Geometry: final body of the model. Coordinates: model frame, mm. A direction names the side the tool comes from. Coordinates: 2 decimals unless noted, no trailing zeros. One line per item, written item: value.
```python
from build123d import *

# Parameters (mm, degrees)
F1_DEPTH = 18
F3_D     = 3
F3_DEPTH = 17.5
F3_TIP   = 0.9012909285
F5_D     = 3
F5_DEPTH = 17.5
F5_TIP   = 0.9012909285
F7_D     = 3
F7_DEPTH = 17.5
F7_TIP   = 0.9012909285


with BuildPart() as f1:
    # F0 (on Top) → F1 (new body)
    with BuildSketch(Plane.XY):
        Polygon((65, 65), (55, 65), (-55, 65), (-65, 65), (-65, 55), (-65, -55), (-65, -65), (-55, -65), (55, -65), (65, -65), (65, -55), (65, 55), align=None)
    extrude(amount=F1_DEPTH)

    # F3
    with Locations(Plane.XZ.offset(65)):
        with Locations((0, 9)):
            Hole(F3_D / 2, depth=F3_DEPTH)
            with Locations((0, 0, -(F3_DEPTH + F3_TIP / 2))):  # 118° drill point
                Cone(0, F3_D / 2, F3_TIP, mode=Mode.SUBTRACT)

    # F5
    with Locations(Plane.YZ.offset(65)):
        with Locations((42.5, 9)):
            Hole(F5_D / 2, depth=F5_DEPTH)
            with Locations((0, 0, -(F5_DEPTH + F5_TIP / 2))):  # 118° drill point
                Cone(0, F5_D / 2, F5_TIP, mode=Mode.SUBTRACT)

    # F7
    with Locations(Plane(origin=(-65, 0, 0), x_dir=(0, -1, 0), z_dir=(-1, 0, 0))):
        with Locations((-42.5, 9)):
            Hole(F7_D / 2, depth=F7_DEPTH)
            with Locations((0, 0, -(F7_DEPTH + F7_TIP / 2))):  # 118° drill point
                Cone(0, F7_D / 2, F7_TIP, mode=Mode.SUBTRACT)


solid = f1.part
```
(1) Line query: line 1 (Z direction, x = -58.5, y = 42.5); line 2 (X direction, y = -61.5, z = 9); line 3 (Y direction, x = 51, z = 8.25). Output: solid intervals per line, ascending. Write a range as [from, to].
Responses:
line 1: z = [0, 7.5], [10.5, 18]
line 2: x = [-65, -1.5], [1.5, 65]
line 3: y = [-65, 41.2], [43.8, 65]
(2) Pull-direction query (Z, two-part tool) for faces 1 (the cylindrical face through (56, 44, 9)), 2 (the flat face through (-1, 1, 0)), 3 (the flat face through (65, -1, 9)); classes: released by +Z, released by -Z, zero draft, split by the parting line, or undercut.
Responses:
face 1: undercut
face 2: released by -Z
face 3: zero draft
(3) First-contact query: pin 1 (1 mm diameter, centred on x = 35.5, y = 33, fed in from -Z); pin 2 (2.5 mm diameter, centred on y = 42.5, z = 9, fed in from -X). Flat tips, straight axial feed; report the tip coordinate or a pass-through.
Responses:
pin 1: stops at z = 0
pin 2: stops at x = -47.35
(4) Reachability of faces 4 (the cylindrical face through (-56.1, 41.3, 8.1)), 5 (the flat face through (-1, -65, 11)), 6 (the cylindrical face through (0.325, -56.128, 7.536)) from +Z, -Z, +X, -X, +Y, -Y: full face, straight path, thin tool, end or side. Return the list, or none.
Responses:
face 4: -X
face 5: +Z, -Z, +X, -X, -Y
face 6: -Y
